from build123d import *

# Parameters (mm, degrees)
SKETCH_1_W                = 594
SKETCH_1_H                = 418
EXTRUDE_1_DEPTH           = 205
SKETCH_2_W                = 576
SKETCH_2_H                = 398
CUT_EXTRUDE_1_DEPTH       = 418.031173895
HOLE_WIZARD_3_0_3_1_D     = 3
HOLE_WIZARD_3_0_3_1_DEPTH = 14.098709071
HOLE_WIZARD_3_0_3_1_TIP   = 0.901290929
CHAMFER_1_SIZE            = 20


with BuildPart() as part:
    # Эскиз1 → Бобышка-Вытянуть1 (new body)
    with BuildSketch(Plane(origin=(0, 0, -205), x_dir=(-1, 0, 0), z_dir=(0, 0, -1))):
        Rectangle(SKETCH_1_W, SKETCH_1_H)
    extrude(amount=-EXTRUDE_1_DEPTH)

    # Эскиз2 → Вырез-Вытянуть1 (cut, through all)
    with BuildSketch(Plane.XY):
        Rectangle(SKETCH_2_W, SKETCH_2_H)
    extrude(amount=-CUT_EXTRUDE_1_DEPTH, mode=Mode.SUBTRACT)

    # Диаметр отверстия Ø3.0 (3)1
    with Locations(Plane.XY):
        with Locations((-293, -169), (-293, -129), (-258, 204), (-293, 169), (-293, 129), (-218, 204), (-258, -204), (-218, -204)):
            Hole(HOLE_WIZARD_3_0_3_1_D / 2, depth=HOLE_WIZARD_3_0_3_1_DEPTH)
            with Locations((0, 0, -(HOLE_WIZARD_3_0_3_1_DEPTH + HOLE_WIZARD_3_0_3_1_TIP / 2))):  # 118° drill point
                Cone(0, HOLE_WIZARD_3_0_3_1_D / 2, HOLE_WIZARD_3_0_3_1_TIP, mode=Mode.SUBTRACT)

    # Фаска1
    chamfer_1_edges = [part.edges().sort_by_distance(p)[0] for p in [
        (288, 199, -102.5),
        (288, -199, -102.5),
        (-288, -199, -102.5),
        (-288, 199, -102.5),
    ]]
    chamfer(chamfer_1_edges, length=CHAMFER_1_SIZE)


solid = part.part
Here's how the part is built. I have some questions about the finished solid (model axes, mm). A direction names the side the tool comes from. Coordinates: 2 decimals unless noted, no trailing zeros. Order: outer loops, then holes, each group sorted by start corner. A loop starts at its lowest first (then second) coordinate and runs counter-clockwise, first axis right, second up. Notation, with made-up numbers: M 45,71.5 L 49,71.5 A26 ccw 49,109.5 Z; hole C 63.5,12 d3. An arc over 180 degrees is marked long. Answer as CSV lines item,"result".
Item 1: If I drill on line 1 (Y direction, x = -218, z = -9.5); line 2 (Y direction, x = -293, z = -3); line 3 (X direction, y = 204, z = -10), over which ranges is the centre line in solid material (lowest first)?
Results found:
line 1,"-209 to -205.5, -202.5 to -199, 199 to 202.5, 205.5 to 209"
line 2,"-209 to -170.5, -167.5 to -130.5, -127.5 to 127.5, 130.5 to 167.5, 170.5 to 209"
line 3,"-297 to -259.5, -256.5 to -219.5, -216.5 to 297"
Item 2: For pin 1 (2.5 mm diameter, centred on x = -258, y = -204, fed in from +Z), with a flat end and sliding along its axis, tell me the tip position at first contact or that it passes through.
Results found:
pin 1,"z = -14.25"
Item 3: Imagine slicing it at C-C on x = 78.5. Write out the boundary of the cut face in (y, z).
Results found:
outline,"M -209,-205 L -199,-205 L -199,0 L -209,0 Z; M 199,-205 L 209,-205 L 209,0 L 199,0 Z"
Item 4: On a 3-axis mill with a long thin cutter (end or side, diameter ignored), from which of +Z, -Z, +X, -X, +Y, -Y can I reach the whole of each face in a straight line? I mean faces 1 (the face through (-288, -3, -101)), 2 (the face through (4, -209, -104)). Say none if no direction works.
Results found:
face 1,"+Z, -Z"
face 2,"+Z, -Z, +X, -X, -Y"
Item 5: Imagine slicing it at A-A on y = -7.5. Write out the boundary of the cut face in (x, z), plus the area to 3 significant figures.
Results found:
outline,"M -297,-205 L -288,-205 L -288,0 L -297,0 Z; M 288,-205 L 297,-205 L 297,0 L 288,0 Z"
area,"3,690 mm2"
Item 6: We'd pull the mould along X, two halves only. Please class faces 3 (the face through (297, -3, -104)), 4 (the face through (1, 202, 0)), 5 (the face through (-4, -199, -101)): +X half, -X half, draft (parallel to the pull), parting line (faces both ways), or undercut.
Results found:
face 3,"+X half"
face 4,"draft"
face 5,"undercut"
Item 7: Imagine slicing it at B-B on z = -122. Write out the boundary of the cut face in (x, y).
Results found:
outline,"M -297,-209 L 297,-209 L 297,209 L -297,209 Z; hole M -288,-179 L -268,-199 L 268,-199 L 288,-179 L 288,179 L 268,199 L -268,199 L -288,179 Z"
